Could you check a few things on this model? Use its own coordinates, in mm. A direction names the side the tool comes from. Coordinates: 2 decimals unless noted, no trailing zeros. Loops run counter-clockwise (first coordinate to the right, second up) from the corner with the lowest first, then second, coordinate; pieces in that order, holes last. Notation, with made-up numbers: (28.5, -4) -> (79.5, -4) arc R23 ccw to (79.5, 27) -> close; hole circle Ø3 at (-28.75, -12). An arc over 180 degrees is marked (long way). One line per question, with ' | ' between items.
```python
from build123d import *

# Parameters (mm, degrees)
F0_W     = 136.54275
F0_H     = 78.149304
F1_DEPTH = 50.8
F2_W     = 31.127811
F2_H     = 59.488708
F3_DEPTH = 94.488


with BuildPart() as f1:
    # F0 (on Front) → F1 (new body)
    with BuildSketch(Plane.XZ):
        Rectangle(F0_W, F0_H)
    extrude(amount=F1_DEPTH)

    # F2 (on face) → F3 (cut)
    with BuildSketch(Plane.YZ.offset(68.271375)):
        with Locations((-24.863321, 2.305764)):
            Rectangle(F2_W, F2_H)
    extrude(amount=-F3_DEPTH, mode=Mode.SUBTRACT)


solid = f1.part
```
Q1. Imagine slicing it at A-A on x = -11.5. Write out the boundary of the cut face in (y, z), plus the area to 3 significant figures.
Values follow:
outline: (-50.8, -39.07) -> (0, -39.07) -> (0, 39.07) -> (-50.8, 39.07) -> close; hole (-40.43, -27.44) -> (-9.3, -27.44) -> (-9.3, 32.05) -> (-40.43, 32.05) -> close | area: 2,120 mm2
Q2. For pin 1 (4 mm diameter, centred on x = -23, z = -13, fed in from +Y); pin 2 (25 mm diameter, centred on y = -22.5, z = -0.5, fed in from +X), each with a flat end and sliding along its axis, tell me the tip position at first contact or that it passes through.
Values follow:
pin 1: stops at y = 0 | pin 2: stops at x = -26.22
Q3. We'd pull the mould along Y, two halves only. Please class faces 1 (the face through (-1, -50.8, 1)), 2 (the face through (22, -40.427, 2)), 3 (the face through (-68.271, -25, -1)): released by +Y, released by -Y, zero draft, split by the parting line, or undercut.
Values follow:
face 1: released by -Y | face 2: undercut | face 3: zero draft
Q4. Imagine slicing it at C-C on y = -19. Write out the boundary of the cut face in (x, z).
Values follow:
outline: (-68.27, -39.07) -> (68.27, -39.07) -> (68.27, -27.44) -> (-26.22, -27.44) -> (-26.22, 32.05) -> (68.27, 32.05) -> (68.27, 39.07) -> (-68.27, 39.07) -> close
Q5. Please list where these lines run through material, in increasing order: L1, parallel to Y at x = 36, z = 5.5; L2, parallel to Z at x = -2, y = -15; L3, parallel to X at y = -21.5, z = 28. Write a range as [from, to].
Values follow:
L1: y = [-50.8, -40.43], [-9.3, 0] | L2: z = [-39.07, -27.44], [32.05, 39.07] | L3: x = [-68.27, -26.22]
Q6. For faces 4 (the face through (-1, -25, 39.075)), 5 (the face through (-26.217, -25, 3)), which set-ups out of +Z, -Z, +X, -X, +Y, -Y let a thin tool reach every point of the face, with its end or its side?
Values follow:
face 4: +Z, +X, -X, +Y, -Y | face 5: +X
Q7. Imagine slicing it at B-B on z = -17. Write out the boundary of the cut face in (x, y), plus the area to 3 significant figures.
Values follow:
outline: (-68.27, -50.8) -> (68.27, -50.8) -> (68.27, -40.43) -> (-26.22, -40.43) -> (-26.22, -9.3) -> (68.27, -9.3) -> (68.27, 0) -> (-68.27, 0) -> close | area: 4,000 mm2
